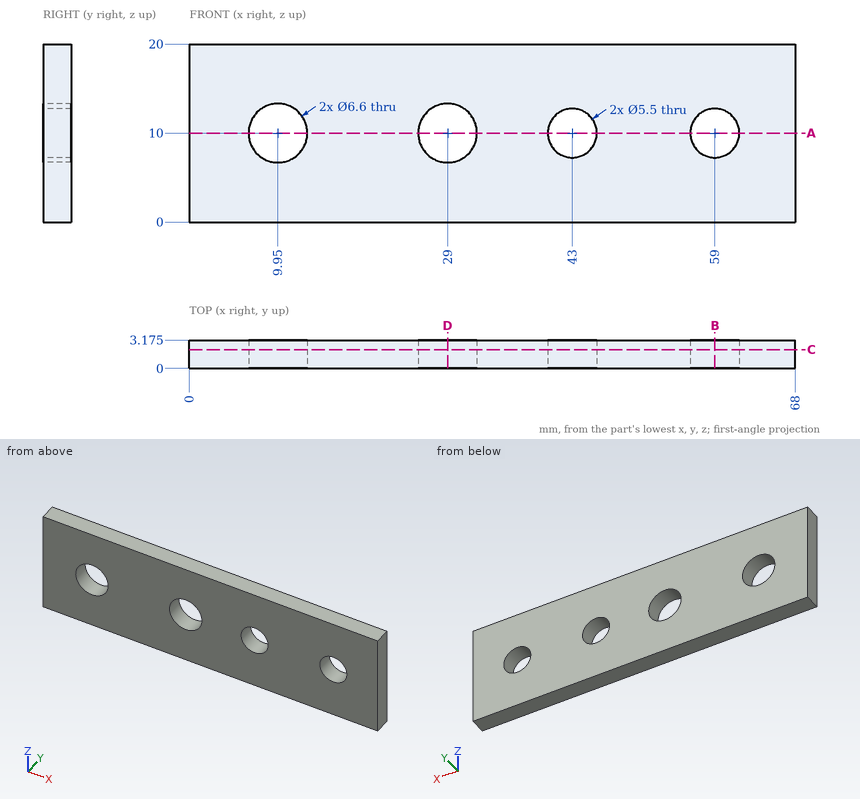
Source: three-view drawing plus pictorial views. Frame: mm from the lowest corner of the part. Round coordinates to 2 decimals unless told otherwise and drop trailing zeros. Loops run counter-clockwise (first coordinate to the right, second up) from the corner with the lowest first, then second, coordinate; pieces in that order, holes last.
Q1. Section C-C, the plane y = 2.1. Return loops of the section in (x, z).
Q2. Ray query, line 1 (X direction, y = 1.2, z = 10); line 2 (Z direction, x = 10, y = 1.5); line 3 (X direction, y = 2.25, z = 9). Return the intervals inside material, ascending.
Q3. Section B-B, the plane x = 59. Return loops of the section in (y, z) (3 decimals).
Q4. Section D-D, the plane x = 29. Return loops of the section in (y, z) (3 decimals), plus the area to 3 significant figures.
Q5. Section A-A, the plane z = 10. Return loops of the section in (x, y) (3 decimals).
Solutions:
1. outline: (0, 0) - (68, 0) - (68, 20) - (0, 20) - close; hole circle Ø6.6 at (9.95, 10); hole circle Ø6.6 at (29, 10); hole circle Ø5.5 at (43, 10); hole circle Ø5.5 at (59, 10)
2. line 1: x = 0 to 6.65, 13.25 to 25.7, 32.3 to 40.25, 45.75 to 56.25, 61.75 to 68
2. line 2: z = 0 to 6.7, 13.3 to 20
2. line 3: x = 0 to 6.81, 13.09 to 25.86, 32.14 to 40.44, 45.56 to 56.44, 61.56 to 68
3. outline: (0, 0) - (3.175, 0) - (3.175, 7.25) - (0, 7.25) - close; (0, 12.75) - (3.175, 12.75) - (3.175, 20) - (0, 20) - close
4. outline: (0, 0) - (3.175, 0) - (3.175, 6.7) - (0, 6.7) - close; (0, 13.3) - (3.175, 13.3) - (3.175, 20) - (0, 20) - close
4. area: 42.5 mm2
5. outline: (0, 0) - (6.65, 0) - (6.65, 3.175) - (0, 3.175) - close; (13.25, 0) - (25.7, 0) - (25.7, 3.175) - (13.25, 3.175) - close; (32.3, 0) - (40.25, 0) - (40.25, 3.175) - (32.3, 3.175) - close; (45.75, 0) - (56.25, 0) - (56.25, 3.175) - (45.75, 3.175) - close; (61.75, 0) - (68, 0) - (68, 3.175) - (61.75, 3.175) - close
